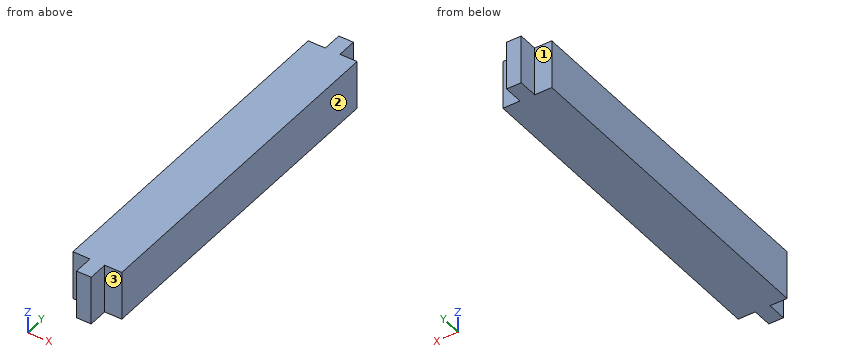
from build123d import *

# Parameters (mm, degrees)
F2_W     = 100
F2_H     = 100
F3_DEPTH = 350
F4_W     = 30
F4_H     = 100
F5_DEPTH = 40


# Not quite as in the source:
# - a pattern or mirror of a feature is missing from the dataset's text; its kind, count and spacing are read off the source's solid


with BuildPart() as f3:
    # F2 (on Front) → F3 (new body, symmetric)
    with BuildSketch(Plane.XZ):
        Rectangle(F2_W, F2_H)
    extrude(amount=F3_DEPTH, both=True)

    # F4 (on face) → F5 (join)
    with BuildSketch(Plane.XZ.offset(350)):
        Rectangle(F4_W, F4_H)
    f5 = extrude(amount=F5_DEPTH)

    # F5_copies: F5 across plane
    add(f5.mirror(Plane.ZX))


solid = f3.part
Design review of the part built by this model. Coordinates are the model's own, in mm. Face numbers are marked on the shaded views. A direction names the side the tool comes from. Round coordinates to 2 decimals unless told otherwise and drop trailing zeros. Write each loop counter-clockwise with the first axis right and the second up, starting at its lowest first coordinate (ties: lowest second). Pieces come first, ordered by that corner, then holes. Notation, with made-up numbers: (74.5, -32.75) - (109.5, -32.75) arc R26 ccw to (109.5, 2.25) - close; hole circle Ø10 at (-15, 2.5). An arc over 180 degrees is marked (long way). Use a Markdown table: item, result. Add a question column.
1. We need section A-A (z = 22). State the section outline as (x, y) points, then the cut area to 3 significant figures.
2. Clearance check with flat-ended pins moving along their axes: pin 1 (1 mm diameter, centred on x = -37, z = -38, fed in from +Y); pin 2 (10.5 mm diameter, centred on x = 28.5, z = 23, fed in from -Y); pin 3 (12 mm diameter, centred on y = 380, z = -24, fed in from +X). State where each tip first meets the part, or that it passes through.
3. Wall thickness on probe 1 along Y at (x, z) = (-22, -0.5): over which ranges is the line inside the solid? List them lowest first.
4. We need section B-B (x = 22). State the section outline as (y, z) points, then the cut area to 3 significant figures.
5. For the marked faces 1, 2 and 3, list the 3-axis set-ups (+Z, -Z, +X, -X, +Y, -Y) from which the entire face can be reached by the end or side of a thin tool; tool diameter is ignored.
Output:
| question | item | result |
|---|---|---|
| 1 | outline | (-50, -350) - (-15, -350) - (-15, -390) - (15, -390) - (15, -350) - (50, -350) - (50, 350) - (15, 350) - (15, 390) - (-15, 390) - (-15, 350) - (-50, 350) - close |
| 1 | area | 72,400 mm2 |
| 2 | pin 1 | stops at y = 350 |
| 2 | pin 2 | stops at y = -350 |
| 2 | pin 3 | stops at x = 15 |
| 3 | probe 1 | y = -350 to 350 |
| 4 | outline | (-350, -50) - (350, -50) - (350, 50) - (-350, 50) - close |
| 4 | area | 70,000 mm2 |
| 5 | face 1 | +Z, -Z, -X, +Y |
| 5 | face 2 | +Z, -Z, +X, +Y, -Y |
| 5 | face 3 | +Z, -Z, +X, -Y |
